Job drawing, mm, ordinate dimensions from the low corner. One solid piece. A direction names the side the tool comes from. Round coordinates to 2 decimals unless told otherwise and drop trailing zeros. Write each loop counter-clockwise with the first axis right and the second up, starting at its lowest first coordinate (ties: lowest second). Pieces come first, ordered by that corner, then holes. Notation, with made-up numbers: M 72,-11.5 L 103,-11.5 A19 cw 103,24.5 Z; hole C 54,-39 d10. An arc over 180 degrees is marked long. Write each question's results on one line, items separated by ' | '. Start each with the question number.
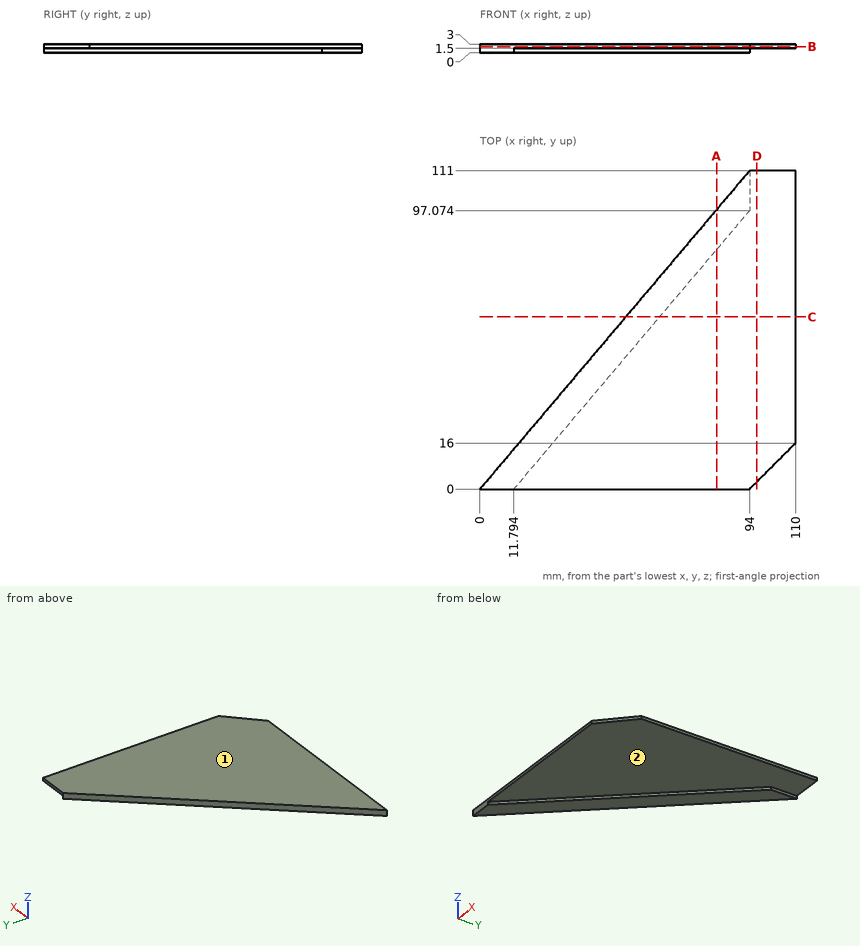
1) Saw through at A-A, the plane x = 82.5. Write the cut outline in (y, z), plus the area to 3 significant figures.
2) Wall check: line 1 along Z through (x, y) = (84.5, 34.5); line 2 along X through (y, z) = (27.5, 2); line 3 along Y through (x, z) = (18.5, 0.8) (1 decimal). Give the ranges that are in metal, low to high. Write a range as from..to.
3) Drop a flat-ended pin along its axis: pin 1 Ø1.6 at (y, z) = (104, 0.5) entering from +X. Give the stop position or say it passes through.
4) Saw through at C-C, the plane y = 60. Write the cut outline in (x, z) (1 decimal).
5) 3-axis set-ups, long thin cutter, end or side, ignore diameter. For the marked faces 1 and 2: which of +Z, -Z, +X, -X, +Y, -Y reach the whole face in a straight line?
6) Saw through at B-B, the plane z = 2.1. Write the cut outline in (x, y).
7) Saw through at D-D, the plane x = 96.5. Write the cut outline in (y, z), plus the area to 3 significant figures.
Filled sheet:
1) outline: M 0,1.5 L 83.49,1.5 L 83.49,0 L 97.42,0 L 97.42,3 L 0,3 Z | area: 167 mm^2
2) line 1: z = 1.5..3 | line 2: x = 23.29..110 | line 3: y = 7.9..21.8
3) pin 1: stops at x = 94
4) outline: M 50.8,0 L 62.6,0 L 62.6,1.5 L 110,1.5 L 110,3 L 50.8,3 Z
5) face 1: +Z, +X, -X, +Y, -Y | face 2: -Z, +X, -Y
6) outline: M 0,0 L 94,0 L 110,16 L 110,111 L 94,111 Z
7) outline: M 2.5,1.5 L 111,1.5 L 111,3 L 2.5,3 Z | area: 163 mm^2
